from build123d import *

# Parameters (mm, degrees)
SKETCH_1_R      = 2.55
SKETCH_1_R_2    = 25
SKETCH_1_R_3    = 2.05
SKETCH_1_W      = 2.1
SKETCH_1_H      = 8.1
EXTRUDE_1_DEPTH = 2


with BuildPart() as part:
    # 草图1 → 凸台-拉伸1 (new body)
    with BuildSketch(Plane.XY):
        Polygon((-52.9, 53.883164809), (-52.9, -50.790000001), (52.9, -50.790000001), (52.9, 53.883164809), (8, 79.569735886), (8, 90.5), (28, 90.5), (28, 106.5), (-28, 106.5), (-28, 90.5), (-8, 90.5), (-8, 79.569735886), align=None)
        with Locations((-23.57, 37.07)):
            Circle(SKETCH_1_R, mode=Mode.SUBTRACT)
        with Locations((-23.57, -10.07)):
            Circle(SKETCH_1_R, mode=Mode.SUBTRACT)
        with Locations((23.57, -10.07)):
            Circle(SKETCH_1_R, mode=Mode.SUBTRACT)
        with Locations((23.57, 37.07)):
            Circle(SKETCH_1_R, mode=Mode.SUBTRACT)
        with Locations((0, 13.5)):
            Circle(SKETCH_1_R_2, mode=Mode.SUBTRACT)
        with Locations((0, 60.5)):
            Circle(SKETCH_1_R_3, mode=Mode.SUBTRACT)
        with Locations((33.234018716, 46.734018716)):
            Circle(SKETCH_1_R_3, mode=Mode.SUBTRACT)
        with Locations((33.234018716, -19.734018716)):
            Circle(SKETCH_1_R_3, mode=Mode.SUBTRACT)
        with Locations((0, -33.5)):
            Circle(SKETCH_1_R_3, mode=Mode.SUBTRACT)
        with Locations((-33.234018716, -19.734018716)):
            Circle(SKETCH_1_R_3, mode=Mode.SUBTRACT)
        with Locations((-33.234018716, 46.734018716)):
            Circle(SKETCH_1_R_3, mode=Mode.SUBTRACT)
        with Locations((0, 78.5)):
            Circle(SKETCH_1_R_3, mode=Mode.SUBTRACT)
        with Locations((-20, 98.5)):
            Circle(SKETCH_1_R_3, mode=Mode.SUBTRACT)
        with Locations((20, 98.5)):
            Circle(SKETCH_1_R_3, mode=Mode.SUBTRACT)
        with Locations((-46, -21.5)):
            Circle(SKETCH_1_R_3, mode=Mode.SUBTRACT)
        with Locations((-46, 8.5)):
            Circle(SKETCH_1_R_3, mode=Mode.SUBTRACT)
        with Locations((46, 8.5)):
            Circle(SKETCH_1_R_3, mode=Mode.SUBTRACT)
        with Locations((46, -21.5)):
            Circle(SKETCH_1_R_3, mode=Mode.SUBTRACT)
        with Locations((-46, 38.5)):
            Circle(SKETCH_1_R_3, mode=Mode.SUBTRACT)
        with Locations((46, 38.5)):
            Circle(SKETCH_1_R_3, mode=Mode.SUBTRACT)
        with Locations((-46, -36.5)):
            Rectangle(SKETCH_1_W, SKETCH_1_H, mode=Mode.SUBTRACT)
        with Locations((-46, -6.5)):
            Rectangle(SKETCH_1_W, SKETCH_1_H, mode=Mode.SUBTRACT)
        with Locations((-46, 23.5)):
            Rectangle(SKETCH_1_W, SKETCH_1_H, mode=Mode.SUBTRACT)
        with Locations((46, 23.5)):
            Rectangle(SKETCH_1_W, SKETCH_1_H, mode=Mode.SUBTRACT)
        with Locations((46, -6.5)):
            Rectangle(SKETCH_1_W, SKETCH_1_H, mode=Mode.SUBTRACT)
        with Locations((46, -36.5)):
            Rectangle(SKETCH_1_W, SKETCH_1_H, mode=Mode.SUBTRACT)
    extrude(amount=EXTRUDE_1_DEPTH)


solid = part.part
Verification items for the finished model (mm, model axes). Coordinates: 2 decimals unless noted, no trailing zeros. Order: outer loops, then holes, each group sorted by start corner. A loop starts at its lowest first (then second) coordinate and runs counter-clockwise, first axis right, second up. Notation, with made-up numbers: (31, 37) -> (75, 37) arc R30 cw to (75, 61) -> close; hole circle Ø9 at (3.25, -36.75). An arc over 180 degrees is marked (long way). Put each result on its own line as item: value. Start each with the question number.
1. Cross-section at C-C, the plane y = 60.5. Record the boundary of the cut face in (x, z).
2. Cross-section at B-B, the plane x = 0. Record the boundary of the cut face in (y, z).
3. Mould release check, pull along X, two halves, no side actions. Record for faces 1 (the cylindrical face through (-21.14, -9.3, 0.99)), 2 (the flat face through (30.76, 66.55, 0.99)), 3 (the cylindrical face through (31.607, 45.487, 0.986)): released by +X, released by -X, zero draft, split by the parting line, or undercut.
4. Cross-section at A-A, the plane y = 98.5. Record the boundary of the cut face in (x, z), then the cut area to 3 significant figures.
5. Go/stop test with a flat-tipped pin: pin 1 Ø0.6 at (x, z) = (-46.5, 1) entering from +Y. Record where the tip stops, or that it passes through.
6. Cross-section at D-D, the plane z = 1.05. Count the separate pieces of the cut face and the enclosed holes in it, then the cut area to 3 significant figures.
7. Material ranges on L1, parallel to X at y = -39, z = 0.8; L2, parallel to X at y = 22, z = 1.5; L3, parallel to Y at x = -20.5, z = 0.2, recorded low to high. Write a range as [from, to].
Computed:
1. outline: (-41.33, 0) -> (-2.05, 0) -> (-2.05, 2) -> (-41.33, 2) -> close; (2.05, 0) -> (41.33, 0) -> (41.33, 2) -> (2.05, 2) -> close
2. outline: (-50.79, 0) -> (-35.55, 0) -> (-35.55, 2) -> (-50.79, 2) -> close; (-31.45, 0) -> (-11.5, 0) -> (-11.5, 2) -> (-31.45, 2) -> close; (38.5, 0) -> (58.45, 0) -> (58.45, 2) -> (38.5, 2) -> close; (62.55, 0) -> (76.45, 0) -> (76.45, 2) -> (62.55, 2) -> close; (80.55, 0) -> (106.5, 0) -> (106.5, 2) -> (80.55, 2) -> close
3. face 1: undercut
3. face 2: released by +X
3. face 3: undercut
4. outline: (-28, 0) -> (-22.05, 0) -> (-22.05, 2) -> (-28, 2) -> close; (-17.95, 0) -> (17.95, 0) -> (17.95, 2) -> (-17.95, 2) -> close; (22.05, 0) -> (28, 0) -> (28, 2) -> (22.05, 2) -> close
4. area: 95.6 mm2
5. pin 1: y = 57.72
6. separate pieces: 1
6. enclosed holes: 26
6. area: 11,400 mm2
7. L1: [-52.9, -47.05], [-44.95, 44.95], [47.05, 52.9]
7. L2: [-52.9, -47.05], [-44.95, -23.51], [23.51, 44.95], [47.05, 52.9]
7. L3: [-50.79, -0.81], [27.81, 72.42], [90.5, 96.51], [100.49, 106.5]
